Input: part model. Units: mm. Frame: model coordinates. A direction names the side the tool comes from. Give positions to 0.01 mm unless a question says otherwise; leave off trailing zeros. Write each loop counter-clockwise with the first axis right and the second up, starting at its lowest first coordinate (ties: lowest second). Pieces come first, ordered by that corner, then holes.
```python
from build123d import *

# Parameters (mm, degrees)
CROQUIS1_W              = 69.85
CROQUIS1_H              = 76.2
EXTRUIR1_DEPTH          = 14.2875
CROQUIS2_R              = 7.9375
CROQUIS2_R_2            = 7.14375
EXTRUIR2_DEPTH          = 4
CROQUIS3_R              = 7.14375
CROQUIS3_R_2            = 3.96875
EXTRUIR3_DEPTH          = 3.5
CROQUIS4_R              = 3.96875
EXTRUIR4_DEPTH          = 25.4
CROQUIS5_W              = 19.05
CROQUIS5_H              = 1.5875
EXTRUIR5_DEPTH          = 3.96875
TALADRO_ROSCADO_10_32_D = 4.0386
CROQUIS7_R              = 8.89
EXTRUIR6_DEPTH          = 0.5
REDONDEO1_R             = 5.08
EXTRUIR7_START          = 3
CROQUIS8_R              = 10
CROQUIS8_R_2            = 7.14375
EXTRUIR7_DEPTH          = 3
EXTRUIR8_START          = 2.5
CROQUIS9_R              = 7.14375
CROQUIS9_R_2            = 3.96875
EXTRUIR8_DEPTH          = 2.5
EXTRUIR9_START          = 3
CROQUIS10_R             = 3.96875
EXTRUIR9_DEPTH          = 3
ENVOLVER1_DEPTH         = 0.5
REDONDEO3_R             = 1.27
CROQUIS15_R             = 7.9375
EXTRUIR13_DEPTH         = 3.175
EXTRUIR14_DEPTH         = 4
FILLET1_R               = 0.762
CHAMFER1_SIZE           = 0.9525


with BuildPart() as part:
    # Croquis1 → Extruir1 (new body)
    with BuildSketch(Plane.XY):
        Rectangle(CROQUIS1_W, CROQUIS1_H)
    extrude(amount=EXTRUIR1_DEPTH)

    # Croquis2 → Extruir2 (add)
    with BuildSketch(Plane.XY.offset(14.2875)):
        with Locations(Location((0, 14.2875, 0), (0, 0, 180))):
            Circle(CROQUIS2_R)
        with Locations((0, 14.2875)):
            Circle(CROQUIS2_R_2, mode=Mode.SUBTRACT)
    extrude(amount=EXTRUIR2_DEPTH)

    # Croquis3 → Extruir3 (add)
    with BuildSketch(Plane.XY.offset(14.2875)):
        with Locations((0, 14.2875)):
            Circle(CROQUIS3_R)
        with Locations((0, 14.2875)):
            Circle(CROQUIS3_R_2, mode=Mode.SUBTRACT)
    extrude(amount=EXTRUIR3_DEPTH)

    # Croquis4 → Extruir4 (add)
    with BuildSketch(Plane.XY.offset(14.2875)):
        with Locations((0, 14.2875)):
            Circle(CROQUIS4_R)
    extrude(amount=EXTRUIR4_DEPTH)

    # Croquis5 → Extruir5 (cut, symmetric)
    with BuildSketch(Plane(origin=(0, 0, 0), x_dir=(0, 0, -1), z_dir=(1, 0, 0))):
        with Locations((-30.1625, 17.4625)):
            Rectangle(CROQUIS5_W, CROQUIS5_H)
    extrude(amount=EXTRUIR5_DEPTH, both=True, mode=Mode.SUBTRACT)

    # Taladro roscado #10-32 (through all)
    with Locations(Plane(origin=(30.1625, 31.75, 14.2875), x_dir=(1, 0, 0), z_dir=(0, 0, 1))):
        with Locations((0, 0), (-60.325, 0), (-60.325, -63.5), (0, -63.5)):
            Hole(TALADRO_ROSCADO_10_32_D / 2)

    # Croquis7 → Extruir6 (add)
    with BuildSketch(Plane.XY.offset(14.2875)):
        with Locations(Location((0, -21.2725, 0), (0, 0, 180))):
            Circle(CROQUIS7_R)
    extrude(amount=EXTRUIR6_DEPTH)

    # Cúpula1: read off the stored shape, not the designer's step
    # Cúpula1 outline → Cúpula1 (revolve)
    with BuildSketch(Plane.XZ.offset(21.2725)):
        with BuildLine():
            Line((0, 14.7875), (8.890000011, 14.787499991))
            ThreePointArc((8.890000011, 14.787499991), (4.719976834, 17.144935114), (0, 17.9625))
            Line((0, 17.9625), (0, 14.7875))
        make_face()
    revolve(axis=Axis((0, -21.2725, 0), (0, 0, 1)))

    # Redondeo1
    redondeo1_edges = [part.edges().sort_by_distance(p)[0] for p in [
        (-34.925, 38.1, 7.14375),
        (34.925, 38.1, 7.14375),
        (34.925, -38.1, 7.14375),
        (-34.925, -38.1, 7.14375),
    ]]
    fillet(redondeo1_edges, radius=REDONDEO1_R)

    # Croquis8 → Extruir7 (add)
    with BuildSketch(Plane(origin=(0, 0, 0), x_dir=(-1, 0, 0), z_dir=(0, 0, -1)).offset(EXTRUIR7_START)):
        with Locations((0, 14.2875)):
            Circle(CROQUIS8_R)
        with Locations(Location((0, 14.2875, 0), (0, 0, 180))):
            Circle(CROQUIS8_R_2, mode=Mode.SUBTRACT)
    extrude(amount=-EXTRUIR7_DEPTH)

    # Croquis9 → Extruir8 (add)
    with BuildSketch(Plane(origin=(0, 0, 0), x_dir=(-1, 0, 0), z_dir=(0, 0, -1)).offset(EXTRUIR8_START)):
        with Locations(Location((0, 14.2875, 0), (0, 0, 180))):
            Circle(CROQUIS9_R)
        with Locations(Location((0, 14.2875, 0), (0, 0, 36.869897646))):
            Circle(CROQUIS9_R_2, mode=Mode.SUBTRACT)
    extrude(amount=-EXTRUIR8_DEPTH)

    # Croquis10 → Extruir9 (add)
    with BuildSketch(Plane(origin=(0, 0, 0), x_dir=(-1, 0, 0), z_dir=(0, 0, -1)).offset(EXTRUIR9_START)):
        with Locations(Location((0, 14.2875, 0), (0, 0, 36.869897646))):
            Circle(CROQUIS10_R)
    extrude(amount=-EXTRUIR9_DEPTH)

    # Envolver1: read off the stored shape, not the designer's step
    # Envolver1 outline → Envolver1 (add)
    with BuildSketch(Plane(origin=(0, 0, 0), x_dir=(-1, 0, 0), z_dir=(0, 0, -1))):
        Polygon((-7.459471243, 34.190889413), (-7.513744748, 34.190889413), (-8.072592237, 29.957556079), (-7.690133636, 29.957556079), (-7.285626425, 33.010440695), (-5.751551906, 29.957556079), (-5.665901532, 29.957556079), (-4.137763177, 33.003656507), (-3.732407942, 29.957556079), (-3.350797365, 29.957556079), (-3.913036948, 34.190889413), (-3.968158476, 34.190889413), (-5.711694801, 30.717385139), align=None)
        Polygon((0.204117165, 34.190889413), (-0.337769854, 34.190889413), (-2.102506767, 32.578796731), (-2.102506767, 34.190889413), (-2.482421297, 34.190889413), (-2.482421297, 29.957556079), (-2.102506767, 29.957556079), (-2.102506767, 32.000444701), (-0.139332354, 29.957556079), (0.366937678, 29.957556079), (-1.876084491, 32.291316763), align=None)
        Polygon((5.929971866, 34.190889413), (5.522920584, 34.190889413), (4.111809472, 30.854764947), (2.700698361, 34.190889413), (2.293647079, 34.190889413), (4.08467272, 29.957556079), (4.138946225, 29.957556079), align=None)
        Polygon((8.752194088, 34.190889413), (6.689800925, 34.190889413), (6.689800925, 29.957556079), (7.069715455, 29.957556079), (7.069715455, 32.019949242), (8.752194088, 32.019949242), (8.752194088, 32.454137276), (7.069715455, 32.454137276), (7.069715455, 33.756701379), (8.752194088, 33.756701379), align=None)
    extrude(amount=ENVOLVER1_DEPTH)

    # Redondeo3
    redondeo3_edges = [part.edges().sort_by_distance(p)[0] for p in [
        (0, -38.1, 0),
        (-34.925, 0, 0),
        (0, 38.1, 0),
        (34.925, 0, 0),
        (-33.437102448, 36.612102448, 0),
        (33.437102448, 36.612102448, 0),
        (33.437102448, -36.612102448, 0),
        (-33.437102448, -36.612102448, 0),
    ]]
    fillet(redondeo3_edges, radius=REDONDEO3_R)

    # Croquis15 → Extruir13 (add)
    with BuildSketch(Plane(origin=(0, 0, 0), x_dir=(-1, 0, 0), z_dir=(0, 0, -1))):
        with Locations((0, -21.2725)):
            Circle(CROQUIS15_R)
    extrude(amount=EXTRUIR13_DEPTH)

    # Croquis16 → Extruir14 (add)
    with BuildSketch(Plane(origin=(0, 0, 0), x_dir=(-1, 0, 0), z_dir=(0, 0, -1))):
        with BuildLine():
            Line((-0.783175899, -29.17126837), (-1, -30.74486111))
            ThreePointArc((-1, -30.74486111), (0, -30.7975), (1, -30.74486111))
            Line((1, -30.74486111), (0.783175899, -29.17126837))
            ThreePointArc((0.783175899, -29.17126837), (0, -29.21), (-0.783175899, -29.17126837))
        make_face()
    extrude(amount=EXTRUIR14_DEPTH)

    # Recubrir1: read off the stored shape, not the designer's step
    # Recubrir1: loft between two sections, ruled curve by curve
    recubrir1_from = [
        Edge.make_bspline([(-1.31936525, -16.449712908, -3.175), (8.326208935, -13.810982408, -3.175), (10.964939434, -23.456556593, -3.175), (1.31936525, -26.095287092, -3.175), (-8.326208935, -28.734017592, -3.175), (-10.964939434, -19.088443407, -3.175), (-1.31936525, -16.449712908, -3.175)], [0, 0, 0, 0, 0.5, 0.5, 0.5, 1, 1, 1, 1], 3, [1, 0.333333333, 0.333333333, 1, 0.333333333, 0.333333333, 1]),
    ]
    recubrir1_to = [
        Edge.make_bspline([(-2.957878031, -20.118557821, -4.675), (-0.649993674, -14.202801759, -4.675), (5.265762389, -16.510686116, -4.675), (2.957878031, -22.426442179, -4.675), (0.649993674, -28.342198241, -4.675), (-5.265762389, -26.034313884, -4.675), (-2.957878031, -20.118557821, -4.675)], [0, 0, 0, 0, 0.5, 0.5, 0.5, 1, 1, 1, 1], 3, [1, 0.333333333, 0.333333333, 1, 0.333333333, 0.333333333, 1]),
    ]
    recubrir1 = Solid(Shell([*[Face.make_surface_from_curves(recubrir1_from[k], recubrir1_to[k]) for k in range(1)], Face(Wire(recubrir1_from)), Face(Wire(recubrir1_to))]))
    add(recubrir1)

    # Sketch2 → Revolve1 (revolve)
    with BuildSketch(Plane(origin=(0, 0, 0), x_dir=(0, 0, -1), z_dir=(1, 0, 0)), mode=Mode.PRIVATE) as revolve1_sk:
        Polygon((3.175, -21.2725), (47.3964, -21.2725), (47.3964, -20.1295), (45.974, -20.1295), (45.974, -16.8275), (47.244, -16.8275), (47.244, -16.3195), (43.688, -16.3195), (43.688, -11.684), (42.164, -11.684), (42.164, -7.874), (43.18, -7.874), (43.18, -7.493), (3.175, -7.493), align=None)
    revolve(revolve1_sk.sketch.rotate(Axis((0, -21.2725, -3.175), (0, 0, -1)), 180), axis=Axis((0, -21.2725, -3.175), (0, 0, -1)))

    # Fillet1
    fillet1_edges = [part.edges().sort_by_distance(p)[0] for p in [
        (0, -11.684, -43.688),
        (0, -20.1295, -47.3964),
    ]]
    fillet(fillet1_edges, radius=FILLET1_R)

    # Chamfer1
    chamfer1_edges = [part.edges().sort_by_distance(p)[0] for p in [
        (7.9375, 14.2875, 14.2875),
    ]]
    chamfer(chamfer1_edges, length=CHAMFER1_SIZE)


solid = part.part
```
Item 1: Pin query (flat end, axial travel): pin 1 (6 mm diameter, centred on x = 19, y = -4, fed in from -Z); pin 2 (3 mm diameter, centred on x = -9, y = -1, fed in from +Z); pin 3 (21 mm diameter, centred on x = -16, y = 14.5, fed in from +Z). Return the tip coordinate at first contact, or that it passes through.
Item 2: Ray query, line 1 (Y direction, x = 0, z = -2.8) (1 decimal); line 2 (Z direction, x = -6.5, y = -31) (1 decimal); line 3 (Z direction, x = -21, y = -32.5). Return the intervals inside material, ascending.
Item 3: Section A-A (x = 12). Return loops of the section in (y, z) (1 decimal), and give its area (3 significant figures).
Item 4: Mould query, pull axis Y, two halves, no side actions, for faces 6 (the flat face through (4, -17, -43.688)), 7 (the flat face through (0, -38.1, 8)), 8 (the cylindrical face through (29.23, 29.96, 7.04)). Classes: +Y half, -Y half, draft (parallel to the pull), parting line (faces both ways), or undercut.
Item 5: Section B-B (y = 1.5). Return loops of the section in (x, z) (1 decimal).
Item 6: Set-up query: faces 1 (the flat face through (7, 11, 18.288)), 2 (the flat face through (-34.925, 0, 8)), 3 (the flat face through (6.42, 31.77, -0.5)), 4 (the cylindrical face through (5.13, -33.65, -42.68)), 5 (the cylindrical face through (-0.338, -13.342, -1.565)). Return all of +Z, -Z, +X, -X, +Y, -Y with unobstructed straight access to the full face (end or side cutting, diameter ignored); none if empty.
Item 7: Section C-C (z = -30). Return loops of the section in (x, y).
Solved:
1. pin 1: stops at z = 0
1. pin 2: stops at z = 14.29
1. pin 3: stops at z = 18.29
2. line 1: y = -30.8 to -13.3, 4.3 to 7.1, 10.3 to 18.3, 21.4 to 24.3
2. line 2: z = -42.2 to -3.2, 0 to 14.3
2. line 3: z = 0 to 14.29
3. outline: (-38.1, 1.3) arc R1.3 ccw to (-36.8, 0) - (36.8, 0) arc R1.3 ccw to (38.1, 1.3) - (38.1, 14.3) - (-38.1, 14.3) - close; (-28, -43.2) - (-27.2, -43.2) - (-27.2, -42.2) - (-15.3, -42.2) - (-15.3, -43.2) - (-14.5, -43.2) - (-14.5, -3.2) - (-28, -3.2) - close
3. area: 1,620 mm2
4. face 6: draft
4. face 7: -Y half
4. face 8: undercut
5. outline: (-34.9, 1.3) arc R1.3 ccw to (-33.7, 0) - (33.7, 0) arc R1.3 ccw to (34.9, 1.3) - (34.9, 14.3) - (-34.9, 14.3) - close
6. face 1: +Z
6. face 2: +Z, -Z, -X, +Y, -Y
6. face 3: -Z, +X, -X, +Y
6. face 4: -Z
6. face 5: none
7. outline: circle Ø27.56 at (0, -21.27)
